Build history of the part. All positions in model axes, mm. Round coordinates to 2 decimals unless told otherwise and drop trailing zeros. Loops run counter-clockwise (first coordinate to the right, second up) from the corner with the lowest first, then second, coordinate; pieces in that order, holes last. Notation, with made-up numbers: (-35, 5.25) - (-8, 5.25) arc R23 ccw to (-8, 41.25) - close; hole circle Ø2 at (67.25, 38.25). An arc over 180 degrees is marked (long way). Answer as CSV lines item,"result". Start each with the question number.
Autodesk Inventor part; units mm, degrees
ref_plane "YZ Plane" through (0, 0, 0) normal (1, 0, 0) x (0, 1, 0)
ref_plane "XZ Plane" through (0, 0, 0) normal (0, 1, 0) x (-1, 0, 0)
ref_plane "XY Plane" through (0, 0, 0) normal (0, 0, 1) x (1, 0, 0)
sketch "Sketch1" plane through (0, 0, 0) normal (0, 0, 1) x (1, 0, 0)
  circle A0 centre (0, 0) radius 4
  circle A1 centre (0, 0) radius 12.5
  circle A2 centre (0, 280) radius 4
  circle A3 centre (0, 280) radius 12.5
  line L0 (12.5, 0) -> (12.5, 280)
  line L1 (-12.5, 280) -> (-12.5, 0)
  dimension "d0" = 8
  dimension "d1" = 25
  dimension "d2" = 280
  dimension "d3" = 0
  dimension "d4" = 8
  dimension "d5" = 25
extrude "Extrusion1" add sketch "Sketch1" along normal blind 4
sketch "Sketch2" plane through (0, 0, 4) normal (0, 0, 1) x (1, 0, 0)
  circle A0 centre (0, 0) radius 4
extrude "Extrusion2" add sketch "Sketch2" against normal blind 50
equation "\"d4\" = d0"
equation "\"d5\" = d1"
properties part number "ramie cięgna traction loss"
Q1. Two-plate mould, pull along X, no slides. Class faces 1 (the cylindrical face through (-0.867, -3.905, -22.678)), 2 (the flat face through (0, 142, 4)), 3 (the cylindrical face through (1.846, 283.549, 1.972)): released by +X, released by -X, zero draft, split by the parting line, or undercut.
Q2. Pin check, flat tips, straight feed: pin 1 Ø3 at (x, z) = (3, -34.5) entering from +Y; pin 2 Ø6 at (y, z) = (36.5, -3.5) entering from +X; pin 3 Ø5 at (x, y) = (9.5, 193.5) entering from -Z. Stop position of each tip, or through.
Q3. Band-saw the part on C-C, the plane z = -33.5. List the corners of the cut face in (x, y).
Q4. Band-saw the part on B-B, the plane y = 72. List the corners of the cut face in (x, z), then the cut area to 3 significant figures.
Q5. Wall check: probe 1 along Y at (x, z) = (0, 1.45); probe 2 along X at (y, z) = (280, 1.65); probe 3 along Z at (x, y) = (-10, 72). Give the ranges that are in metal, low to high. Write a range as [from, to].
Q6. Band-saw the part on A-A, the plane x = 0. List the corners of the cut face in (y, z).
Reported:
1,face 1,"split by the parting line"
1,face 2,"zero draft"
1,face 3,"undercut"
2,pin 1,"stops at y = 3.71"
2,pin 2,"passes through"
2,pin 3,"stops at z = 0"
3,outline,"circle Ø8 at (0, 0)"
4,outline,"(-12.5, 0) - (12.5, 0) - (12.5, 4) - (-12.5, 4) - close"
4,area,"100 mm2"
5,probe 1,"y = [-12.5, 276], [284, 292.5]"
5,probe 2,"x = [-12.5, -4], [4, 12.5]"
5,probe 3,"z = [0, 4]"
6,outline,"(-12.5, 0) - (-4, 0) - (-4, -46) - (4, -46) - (4, 0) - (276, 0) - (276, 4) - (-12.5, 4) - close; (284, 0) - (292.5, 0) - (292.5, 4) - (284, 4) - close"
